```python
from build123d import *

# Parameters (mm, degrees)
F1_DEPTH     = 76.2
F2_R         = 17.4749230477
F2_R_2       = 8.76970131
F3_DEPTH     = 50.8
F4_T         = 2.54
F5_T5_DEPTH  = 101.6
F5_T7_DEPTH  = 101.6
F5_T14_ANGLE = 151.9275130641
F5_T16_ANGLE = 208.0724869359


# Not quite as in the source:
# - a fillet or chamfer that OpenCascade refuses, or shapes differently, is made with other operations: its cross-section is extruded or revolved along the edge and cut away or added
# - a shell that OpenCascade refuses in one call is made with other operations: the cavity is built on its own and cut out


with BuildPart() as f1:
    # F0 (on Front) → F1 (new body)
    with BuildSketch(Plane.XZ):
        with BuildLine():
            ThreePointArc((9.2406073139, -36.9624292555), (30.0306271884, -23.4472051782), (38.1, 0))
            ThreePointArc((38.1, 0), (30.0306271884, 23.4472051782), (9.2406073139, 36.9624292555))
            ThreePointArc((9.2406073139, 36.9624292555), (-38.1, 0), (9.2406073139, -36.9624292555))
        make_face()
        with BuildLine():
            ThreePointArc((9.2406073139, 36.9624292555), (30.0306271884, 23.4472051782), (38.1, 0))
            ThreePointArc((38.1, 0), (30.0306271884, -23.4472051782), (9.2406073139, -36.9624292555))
            Line((9.2406073139, -36.9624292555), (107.8070853287, -12.3208097518))
            ThreePointArc((107.8070853287, -12.3208097518), (92.0268828907, 0), (107.8070853287, 12.3208097518))
            Line((107.8070853287, 12.3208097518), (9.2406073139, 36.9624292555))
        make_face()
        with BuildLine():
            ThreePointArc((117.4268828907, 0), (114.7370919535, 7.8157350594), (107.8070853287, 12.3208097518))
            ThreePointArc((107.8070853287, 12.3208097518), (92.0268828907, 0), (107.8070853287, -12.3208097518))
            ThreePointArc((107.8070853287, -12.3208097518), (114.7370919535, -7.8157350594), (117.4268828907, 0))
        make_face()
    extrude(amount=F1_DEPTH)

    # F2 (on face) → F3 (cut)
    with BuildSketch(Plane(origin=(0, 0, 0), x_dir=(-1, 0, 0), z_dir=(0, 1, 0))):
        Circle(F2_R)
        with Locations((-104.7268828907, 0)):
            Circle(F2_R_2)
    extrude(amount=-F3_DEPTH, mode=Mode.SUBTRACT)

    # F4: shell of thickness 2.54, made by hand


with BuildPart() as f4_core1:
    # F4_t2: copy of F1
    add(f1.part)

    # the walls: a layer under each face that stays
    f4_faces = [f4_core1.faces().sort_by_distance(p)[0] for p in [
        (-38.1, -38.1, 0),
        (58.5238463213, -38.1, 24.6416195037),
        (58.5238463213, -38.1, -24.6416195037),
        (39.6634414453, 0, 0),
        (117.4268828907, -38.1, 0),
        (113.4965842007, -25.4, 0),
        (17.4749230477, -25.4, 0),
        (104.7268828907, -50.8, 0),
        (0, -50.8, 0),
    ]]
    thicken(f4_faces, amount=-F4_T, mode=Mode.SUBTRACT)

    # F4_s3 → F4_t4 (revolve, cut)
    with BuildSketch(Plane.XY):
        Polygon((95.9825815807, -50.7746), (93.4171815807, -50.8), (93.4171815807, -53.34), (95.9571815807, -53.34), align=None)
    revolve(axis=Axis((104.7268828907, -50.8, 0), (0, 1, 0)), mode=Mode.SUBTRACT)

    # F4_s5 → F4_t6 (revolve, cut)
    with BuildSketch(Plane.XY):
        Polygon((-17.4495230477, -50.7746), (-20.0149230477, -50.8), (-20.0149230477, -53.34), (-17.4749230477, -53.34), align=None)
    revolve(axis=Axis((0, -50.8, 0), (0, 1, 0)), mode=Mode.SUBTRACT)


with BuildPart() as f1_1:
    add(f1.part)

    # what is left inside the walls is the cavity
    f4_cavity = [f4_core1.part.solids().sort_by_distance(p)[0] for p in [
        (-35.5346, -51.646667, 0),
    ]]
    add(f4_cavity, mode=Mode.SUBTRACT)

    # F5: fillet of radius 6.35 on 5 edges, made by hand

    # F5_s1 → F5_t2 (revolve)
    with BuildSketch(Plane.XY):
        with BuildLine():
            ThreePointArc((95.9571815807, -44.45), (97.8170535202, -48.9401280605), (102.3071815807, -50.8))
            Line((102.3071815807, -50.8), (95.9571815807, -50.8))
            Line((95.9571815807, -50.8), (95.9571815807, -44.45))
        make_face()
    revolve(axis=Axis((104.7268828907, -50.8, 0), (0, 1, 0)))

    # F5_s3 → F5_t4 (revolve)
    with BuildSketch(Plane.XY):
        with BuildLine():
            ThreePointArc((-17.4749230477, -44.45), (-15.6150511082, -48.9401280605), (-11.1249230477, -50.8))
            Line((-11.1249230477, -50.8), (-17.4749230477, -50.8))
            Line((-17.4749230477, -50.8), (-17.4749230477, -44.45))
        make_face()
    revolve(axis=Axis((0, -50.8, 0), (0, 1, 0)))

    # F5_s6 → F5_t5 (cut)
    with BuildSketch(Plane(origin=(98.5664780148, 0, -24.6416195037), x_dir=(0, 1, 0), z_dir=(-0.9701425001, 0, 0.242535625))):
        with BuildLine():
            ThreePointArc((-6.35, -38.1), (-1.8598719395, -36.2401280605), (0, -31.75))
            Line((0, -31.75), (0, -38.1))
            Line((0, -38.1), (-6.35, -38.1))
        make_face()
    extrude(amount=F5_T5_DEPTH, mode=Mode.SUBTRACT)

    # F5_s8 → F5_t7 (cut)
    with BuildSketch(Plane(origin=(0, 0, 0), x_dir=(0, 1, 0), z_dir=(0.9701425001, 0, 0.242535625))):
        with BuildLine():
            ThreePointArc((-6.35, -38.1), (-1.8598719395, -36.2401280605), (0, -31.75))
            Line((0, -31.75), (0, -38.1))
            Line((0, -38.1), (-6.35, -38.1))
        make_face()
    extrude(amount=F5_T7_DEPTH, mode=Mode.SUBTRACT)

    # F5_s9 → F5_t10 (revolve, cut)
    with BuildSketch(Plane.XY):
        with BuildLine():
            ThreePointArc((89.6071815807, 0), (94.0973096412, -1.8598719395), (95.9571815807, -6.35))
            Line((95.9571815807, -6.35), (95.9571815807, 0))
            Line((95.9571815807, 0), (89.6071815807, 0))
        make_face()
    revolve(axis=Axis((104.7268828907, 0, 0), (0, 1, 0)), mode=Mode.SUBTRACT)

    # F5_s11 → F5_t12 (revolve, cut)
    with BuildSketch(Plane.XY):
        with BuildLine():
            ThreePointArc((-23.8249230477, 0), (-19.3347949872, -1.8598719395), (-17.4749230477, -6.35))
            Line((-17.4749230477, -6.35), (-17.4749230477, 0))
            Line((-17.4749230477, 0), (-23.8249230477, 0))
        make_face()
    revolve(axis=Axis((0, 0, 0), (0, 1, 0)), mode=Mode.SUBTRACT)

    # F5_s13 → F5_t14 (revolve, cut)
    with BuildSketch(Plane(origin=(98.5664780148, 0, 24.6416195037), x_dir=(0, 1, 0), z_dir=(-0.9701425001, 0, -0.242535625))):
        with BuildLine():
            ThreePointArc((0, 31.75), (-1.8598719395, 36.2401280605), (-6.35, 38.1))
            Line((-6.35, 38.1), (0, 38.1))
            Line((0, 38.1), (0, 31.75))
        make_face()
    revolve(axis=Axis((104.7268828907, 0, 0), (0, -1, 0)), revolution_arc=F5_T14_ANGLE, mode=Mode.SUBTRACT)

    # F5_s15 → F5_t16 (revolve, cut)
    with BuildSketch(Plane(origin=(0, 0, 0), x_dir=(0, 1, 0), z_dir=(0.9701425001, 0, -0.242535625))):
        with BuildLine():
            ThreePointArc((-6.35, 38.1), (-1.8598719395, 36.2401280605), (0, 31.75))
            Line((0, 31.75), (0, 38.1))
            Line((0, 38.1), (-6.35, 38.1))
        make_face()
    revolve(axis=Axis((0, 0, 0), (0, -1, 0)), revolution_arc=F5_T16_ANGLE, mode=Mode.SUBTRACT)


solid = f1_1.part
```
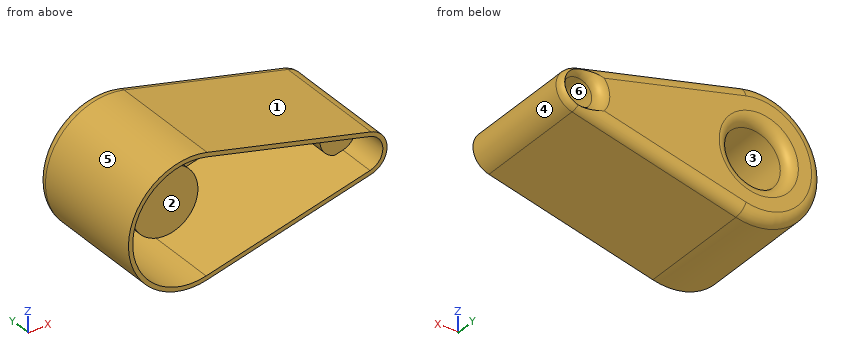
Here's how the part is built. I have some questions about the finished solid (model axes, mm). Face numbers are marked on the shaded views. A direction names the side the tool comes from. Coordinates: 2 decimals unless noted, no trailing zeros. Loops run counter-clockwise (first coordinate to the right, second up) from the corner with the lowest first, then second, coordinate; pieces in that order, holes last. Notation, with made-up numbers: (-9.5, 45) - (23.5, 45) arc R7 cw to (23.5, 51) - close; hole circle Ø6 at (48, -25). An arc over 180 degrees is marked (long way). Return JSON: item names as keys, results as strings. Group by question number.
Item 1: On a 3-axis mill with a long thin cutter (end or side, diameter ignored), from which of +Z, -Z, +X, -X, +Y, -Y can I reach the whole of each face in a straight line? I mean the marked faces 1, 2 and 3. Say none if no direction works.
Item 2: We'd pull the mould along X, two halves only. Please class the marked faces 4, 5 and 6: +X half, -X half, draft (parallel to the pull), parting line (faces both ways), or undercut.
Item 3: If we section it at A-A on y = -33.5: Write out the boundary of the cut face in (x, z), and give its area (3 significant figures).
Item 4: I need wall thicknesses on line 1 (Z direction, x = 0, y = -18.5); line 2 (Y direction, x = 3.5, z = -6); line 3 (Z direction, x = -23.5, y = -28.5). Which ranges of each line are inside material? Lowest first, please. Write a range as from..to.
Item 5: If we section it at B-B on y = -64.5: Write out the boundary of the cut face in (x, z), and give its area (3 significant figures).
Item 6: If we section it at C-C on x = 0: Write out the boundary of the cut face in (y, z), and give its area (4 significant figures).
Item 7: Will these pins go through, and if not, where does the flat tip stop? P1, Ø5, axis at x = 49.5, y = -11.5, coming from the +Z side; P2, Ø5.5, axis at x = 105, z = -1, coming from the +Y side; P3, Ø24.5, axis at x = -2, z = -2.5, coming from the +Y side.
Calculated:
{
 "1": {"face 1": "+Z, +X, +Y, -Y", "face 2": "-Y", "face 3": "+Y"},
 "2": {"face 4": "+X half", "face 5": "parting line", "face 6": "undercut"},
 "3": {"outline": "circle Ø40.03 at (0, 0); (9.24, -36.96) - (107.81, -12.32) arc R12.7 ccw to (107.81, 12.32) - (9.24, 36.96) arc R38.1 ccw (long way) to start; hole circle Ø34.95 at (0, 0); hole (8.62, -34.5) - (102.37, -11.06) arc R11.31 cw to (102.37, 11.06) - (8.62, 34.5) arc R35.56 ccw (long way) to start; hole circle Ø17.54 at (104.73, 0)", "area": "1,350 mm^2"},
 "4": {"line 1": "z = -38.1..-35.56, -20.01..-17.47, 17.47..20.01, 35.56..38.1", "line 2": "y = -53.34..-50.8", "line 3": "z = -29.99..-26.69, 26.69..29.99"},
 "5": {"outline": "(9.24, -36.96) - (107.81, -12.32) arc R12.7 ccw to (107.81, 12.32) - (9.24, 36.96) arc R38.1 ccw (long way) to start; hole (8.62, -34.5) - (107.19, -9.86) arc R10.16 ccw to (107.19, 9.86) - (8.62, 34.5) arc R35.56 ccw (long way) to start", "area": "933 mm^2"},
 "6": {"outline": "(-76.2, -38.1) - (-6.35, -38.1) arc R6.35 ccw to (0, -31.75) - (0, -23.82) arc R6.35 ccw to (-6.35, -17.47) - (-44.45, -17.47) arc R6.35 cw to (-50.8, -11.12) - (-50.8, 11.12) arc R6.35 cw to (-44.45, 17.47) - (-6.35, 17.47) arc R6.35 ccw to (0, 23.82) - (0, 31.75) arc R6.35 ccw to (-6.35, 38.1) - (-76.2, 38.1) - (-76.2, 35.56) - (-2.54, 35.56) - (-2.54, 20.01) - (-53.34, 20.01) - (-53.34, -20.01) - (-2.54, -20.01) - (-2.54, -35.56) - (-76.2, -35.56) - close", "area": "808.5 mm^2"},
 "7": {"P1": "stops at z = 27.52", "P2": "stops at y = -50.65", "P3": "stops at y = -49.1"}
}
